from build123d import *

# Parameters (mm, degrees)
F0_R     = 10
F1_DEPTH = 170
F2_R     = 14
F3_DEPTH = 7
F4_R     = 6


with BuildPart() as f1:
    # F0 (on Front) → F1 (new body)
    with BuildSketch(Plane.XZ):
        Circle(F0_R)
    extrude(amount=-F1_DEPTH)

    # F2 (on Front) → F3 (join)
    with BuildSketch(Plane.XZ):
        Circle(F2_R)
    extrude(amount=F3_DEPTH)

    # F4
    f4_edges = [f1.edges().sort_by_distance(p)[0] for p in [
        (-14, -7, 0),
    ]]
    fillet(f4_edges, radius=F4_R)


solid = f1.part
Here's how the part is built. I have some questions about the finished solid (model axes, mm). A direction names the side the tool comes from. Round coordinates to 2 decimals unless told otherwise and drop trailing zeros. Order: outer loops, then holes, each group sorted by start corner. A loop starts at its lowest first (then second) coordinate and runs counter-clockwise, first axis right, second up. Notation, with made-up numbers: M -34.5,-32.5 L 4.5,-32.5 A19 ccw 4.5,3.5 Z; hole C 43.5,56.5 d2. An arc over 180 degrees is marked long. Return JSON: item names as keys, results as strings. Group by question number.
1. On a 3-axis mill with a long thin cutter (end or side, diameter ignored), from which of +Z, -Z, +X, -X, +Y, -Y can I reach the whole of each face in a straight line? I mean faces 1 (the face through (12.932, -0.493, -5.362)), 2 (the face through (-2.17, 83.81, -9.76)). Say none if no direction works.
2. If we section it at C-C on y = 150: List the corners of the cut face in (x, z) for me, then the cut area to 3 significant figures.
3. Please list where these lines run through material, in increasing order: probe 1 along X at (y, z) = (100, 0.5); probe 2 along Z at (x, y) = (-0.75, 137.5); probe 3 along Z at (x, y) = (-3.5, 57).
4. I'm going to push flat-ended pins straight in: pin 1 Ø5 at (x, z) = (9, 7) entering from -Y; pin 2 Ø10 at (x, y) = (-5, 152.5) entering from -Z; pin 3 Ø8 at (y, z) = (68.5, 3.5) entering from +X. Where does each tip first touch, or does it pass through?
5. If we section it at A-A on z = 0: List the corners of the cut face in (x, y) for me.
6. If we section it at B-B on x = 0: List the corners of the cut face in (y, z) for me.
Reply:
{
 "1": {"face 1": "+Y, -Y", "face 2": "+Y"},
 "2": {"outline": "C 0,0 d20", "area": "314 mm^2"},
 "3": {"probe 1": "-9.99 to 9.99", "probe 2": "-9.97 to 9.97", "probe 3": "-9.37 to 9.37"},
 "4": {"pin 1": "y = -6.93", "pin 2": "z = -10", "pin 3": "x = 10"},
 "5": {"outline": "M -14,-1 A6 ccw -8,-7 L 8,-7 A6 ccw 14,-1 L 14,0 L 10,0 L 10,170 L -10,170 L -10,0 L -14,0 Z"},
 "6": {"outline": "M -7,-8 A6 ccw -1,-14 L 0,-14 L 0,-10 L 170,-10 L 170,10 L 0,10 L 0,14 L -1,14 A6 ccw -7,8 Z"}
}
